from build123d import *

# Parameters (mm, degrees)
SZKIC1_R                                            = 49
SZKIC1_R_2                                          = 25
DODANIE_WYCI_GNI_CIE1_DEPTH                         = 7
POG_BIENIE_STO_KOWE_POD_M5_DIN965_WKR_T_D           = 5.5
POG_BIENIE_STO_KOWE_POD_M5_DIN965_WKR_T_CSINK_D     = 9.2
POG_BIENIE_STO_KOWE_POD_M5_DIN965_WKR_T_CSINK_ANGLE = 90
SZYK_KO_OWY1_COUNT                                  = 6
SZKIC5_R                                            = 3.3
WYTNIJ_WYCI_GNI_CIE1_DEPTH                          = 6


with BuildPart() as part:
    # Szkic1 → Dodanie-wyciągnięcie1 (new body)
    with BuildSketch(Plane.XY):
        Circle(SZKIC1_R)
        Circle(SZKIC1_R_2, mode=Mode.SUBTRACT)
    extrude(amount=DODANIE_WYCI_GNI_CIE1_DEPTH)

    # Pogłębienie stożkowe pod M5 DIN965 Wkręt z łbem płaskim1 (through all)
    with Locations(Plane(origin=(0, 0, 0), x_dir=(-1, 0, 0), z_dir=(0, 0, -1))):
        with Locations((44, 0)):
            pog_bienie_sto_kowe_pod_m5_din965_wkr_t = CounterSinkHole(POG_BIENIE_STO_KOWE_POD_M5_DIN965_WKR_T_D / 2, POG_BIENIE_STO_KOWE_POD_M5_DIN965_WKR_T_CSINK_D / 2, counter_sink_angle=POG_BIENIE_STO_KOWE_POD_M5_DIN965_WKR_T_CSINK_ANGLE)

    # Szyk kołowy1: Pogłębienie stożkowe pod M5 DIN965 Wkręt z łbem płaskim1 ×6 about axis
    szyk_ko_owy1_axis = Axis((0, 0, 0), (0, 0, 1))
    for i in range(1, SZYK_KO_OWY1_COUNT):
        add(pog_bienie_sto_kowe_pod_m5_din965_wkr_t.rotate(szyk_ko_owy1_axis, i * 360 / SZYK_KO_OWY1_COUNT), mode=Mode.SUBTRACT)

    # Szkic5 → Wytnij-wyciągnięcie1 (cut)
    with BuildSketch(Plane(origin=(0, 0, 0), x_dir=(-1, 0, 0), z_dir=(0, 0, -1))):
        with Locations((23.6, 23.6)):
            Circle(SZKIC5_R)
        with Locations((23.6, -23.6)):
            Circle(SZKIC5_R)
        with Locations((-23.6, 23.6)):
            Circle(SZKIC5_R)
        with Locations((-23.6, -23.6)):
            Circle(SZKIC5_R)
    extrude(amount=-WYTNIJ_WYCI_GNI_CIE1_DEPTH, mode=Mode.SUBTRACT)


solid = part.part
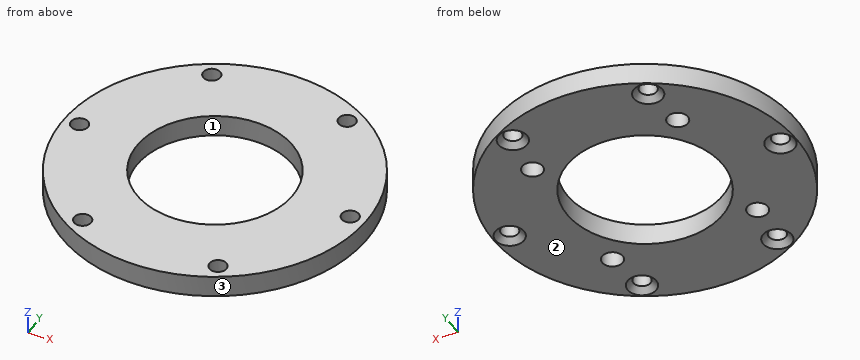
CAD build for the part. Positions are in the model's coordinates, mm. Face numbers are marked on the shaded views. Round coordinates to 2 decimals unless told otherwise and drop trailing zeros. Write each loop counter-clockwise with the first axis right and the second up, starting at its lowest first coordinate (ties: lowest second). Pieces come first, ordered by that corner, then holes. Notation, with made-up numbers: M -13.5,37.5 L 36.5,37.5 A30 cw 36.5,59.5 Z; hole C -12.75,54.5 d1. An arc over 180 degrees is marked long. Put each result on its own line as item: value. Start each with the question number.
1) Saw through at B-B, the plane x = 0. Write the cut outline in (y, z), and give its area (3 significant figures).
2) Saw through at A-A, the plane y = 0. Write the cut outline in (x, z).
3) Drill centre lines: probe 1 along X at (y, z) = (40.5, 3.5); probe 2 along Y at (x, z) = (-22, 5.15); probe 3 along X at (y, z) = (39, 5.5). Where is each one in solid material? Low to high. Write a range as [from, to].
4) Pin check, flat tips, straight feed: pin 1 Ø4 at (x, y) = (-23.6, 23.6) entering from -Z; pin 2 Ø5 at (x, y) = (22, -38.11) entering from +Z; pin 3 Ø9 at (x, y) = (-22, 38.11) entering from -Z; pin 4 Ø1 at (y, z) = (24.5, 3.5) entering from +X. Stop position of each tip, or through.
5) Pull direction X, two halves, no side cores. Call the marked faces 1, 2 and 3: pulls with the +X half, pulls with the -X half, needs draft (parallel to the pull), parting line crosses it, or undercut.
6) Saw through at D-D, the plane x = -22. Write the cut outline in (y, z).
7) Saw through at C-C, the plane y = -23.6. Write the cut outline in (x, z).
Resolved:
1. outline: M -49,0 L -25,0 L -25,7 L -49,7 Z; M 25,0 L 49,0 L 49,7 L 25,7 Z
1. area: 336 mm²
2. outline: M -49,0 L -48.6,0 L -46.75,1.85 L -46.75,7 L -49,7 Z; M -41.25,1.85 L -39.4,0 L -25,0 L -25,7 L -41.25,7 Z; M 25,0 L 39.4,0 L 41.25,1.85 L 41.25,7 L 25,7 Z; M 46.75,1.85 L 48.6,0 L 49,0 L 49,7 L 46.75,7 Z
3. probe 1: [-27.58, -23.35], [-20.65, 20.65], [23.35, 27.58]
3. probe 2: [-43.78, -40.86], [-35.36, -26.49], [-20.71, -11.87], [11.87, 20.71], [26.49, 35.36], [40.86, 43.78]
3. probe 3: [-29.66, -24.6], [-19.4, 19.4], [24.6, 29.66]
4. pin 1: z = 6
4. pin 2: through
4. pin 3: z = 0.1
4. pin 4: x = 42.72
5. face 1: undercut
5. face 2: needs draft
5. face 3: parting line crosses it
6. outline: M -43.78,0 L -42.71,0 L -40.86,1.85 L -40.86,7 L -43.78,7 Z; M -35.36,1.85 L -33.51,0 L -26.49,0 L -26.49,6 L -20.71,6 L -20.71,0 L -11.87,0 L -11.87,7 L -35.36,7 Z; M 11.87,0 L 20.71,0 L 20.71,6 L 26.49,6 L 26.49,0 L 33.51,0 L 35.36,1.85 L 35.36,7 L 11.87,7 Z; M 40.86,1.85 L 42.71,0 L 43.78,0 L 43.78,7 L 40.86,7 Z
7. outline: M -42.94,0 L -26.9,0 L -26.9,6 L -20.3,6 L -20.3,0 L -8.25,0 L -8.25,7 L -42.94,7 Z; M 8.25,0 L 20.3,0 L 20.3,6 L 26.9,6 L 26.9,0 L 42.94,0 L 42.94,7 L 8.25,7 Z
